Verification items for the finished model (mm, model axes). Round coordinates to 2 decimals unless told otherwise and drop trailing zeros. Write each loop counter-clockwise with the first axis right and the second up, starting at its lowest first coordinate (ties: lowest second). Pieces come first, ordered by that corner, then holes. Notation, with made-up numbers: M -38.5,42 L -23.5,42 A30 cw -23.5,64 Z; hole C -24,-8 d7. An arc over 180 degrees is marked long. One line per question, with ' | ' between items. Start each with the question number.
Q1. Thickness scan on line 1 along Y through (x, z) = (0, 2.95); line 2 along Y through (x, z) = (-3.25, 2.7); line 3 along X through (y, z) = (1.75, 3.6). Record the ranges inside material, lowest first. Write a range as from..to.
Q2. Release check for a two-part mould opening along Y. For faces 1 (the face through (-2, 4, 0)), 2 (the face through (-0.867, -3.905, 2.469)), 3 (the face through (-1.19, -5.37, 2.47)) record: released by +Y, released by -Y, zero draft, split by the parting line, or undercut.
Q3. Cross-section at A-A (y = 0). Record the boundary of the cut face in (x, z), then the cut area to 3 significant figures.
Q4. Gauge pin test, flat ends, axial feed: pin 1 (1 mm diameter, centred on y = -3, z = 0.5, fed in from -X); pin 2 (1 mm diameter, centred on y = 1.5, z = 0.5, fed in from +X); pin 3 (2 mm diameter, centred on x = 1, z = 3.5, fed in from -Y); pin 4 (2 mm diameter, centred on x = 0.5, y = -2, fed in from -Z). Record the tip position at first contact, or that the pin passes through.
Q5. Cross-section at C-C (z = 4.15). Record the boundary of the cut face in (x, y), then the cut area to 3 significant figures.
from build123d import *

# Parameters (mm, degrees)
SKETCH1_R           = 5.5
SKETCH1_R_2         = 4
BOSS_EXTRUDE1_DEPTH = 5
FILLET1_R           = 0.3
FILLET2_R           = 0.3
FILLET3_R           = 0.3


with BuildPart() as part:
    # Sketch1 → Boss-Extrude1 (new body)
    with BuildSketch(Plane.XY):
        Circle(SKETCH1_R)
        Circle(SKETCH1_R_2, mode=Mode.SUBTRACT)
    extrude(amount=BOSS_EXTRUDE1_DEPTH)

    # Fillet1
    fillet1_edges = [part.edges().sort_by_distance(p)[0] for p in [
        (-5.5, 0, 0),
    ]]
    fillet(fillet1_edges, radius=FILLET1_R)

    # Fillet2
    fillet2_edges = [part.edges().sort_by_distance(p)[0] for p in [
        (-4, 0, 0),
    ]]
    fillet(fillet2_edges, radius=FILLET2_R)

    # Fillet3
    fillet3_edges = [part.edges().sort_by_distance(p)[0] for p in [
        (-5.5, 0, 5),
        (-4, 0, 5),
    ]]
    fillet(fillet3_edges, radius=FILLET3_R)


solid = part.part
Determined:
1) line 1: y = -5.5..-4, 4..5.5 | line 2: y = -4.44..-2.33, 2.33..4.44 | line 3: x = -5.21..-3.6, 3.6..5.21
2) face 1: zero draft | face 2: undercut | face 3: split by the parting line
3) outline: M -5.5,0.3 A0.3 ccw -5.2,0 L -4.3,0 A0.3 ccw -4,0.3 L -4,4.7 A0.3 ccw -4.3,5 L -5.2,5 A0.3 ccw -5.5,4.7 Z; M 4,0.3 A0.3 ccw 4.3,0 L 5.2,0 A0.3 ccw 5.5,0.3 L 5.5,4.7 A0.3 ccw 5.2,5 L 4.3,5 A0.3 ccw 4,4.7 Z | area: 14.8 mm²
4) pin 1: stops at x = -4.9 | pin 2: stops at x = 5.41 | pin 3: stops at y = -5.5 | pin 4: passes through
5) outline: C 0,0 d11; hole C 0,0 d8 | area: 44.8 mm²
